from build123d import *

# Parameters (mm, degrees)
F1_DEPTH = 25.4
F3_DEPTH = 12.7
F5_DEPTH = 12.7
F7_DEPTH = 12.7


with BuildPart() as f1:
    # F0 (on Top) → F1 (new body)
    with BuildSketch(Plane.XY):
        Polygon((-12.7, 31.75), (0, 31.75), (0, 0), (12.7, 0), (12.7, 31.75), (25.4, 31.75), (25.4, 57.15), (-12.7, 57.15), align=None)
    extrude(amount=F1_DEPTH)

    # F2 (on face) → F3 (cut)
    with BuildSketch(Plane(origin=(-12.7, 0, 0), x_dir=(0, -1, 0), z_dir=(-1, 0, 0))):
        Polygon((-31.75, 25.4), (-44.45, 25.4), (-31.75, 0), align=None)
    extrude(amount=-F3_DEPTH, mode=Mode.SUBTRACT)

    # F4 (on face) → F5 (cut)
    with BuildSketch(Plane.YZ.offset(25.4)):
        Polygon((31.75, 0), (44.45, 25.4), (31.75, 25.4), align=None)
    extrude(amount=-F5_DEPTH, mode=Mode.SUBTRACT)

    # F6 (on face) → F7 (cut)
    with BuildSketch(Plane(origin=(0, 0, 0), x_dir=(0, -1, 0), z_dir=(-1, 0, 0))):
        Polygon((0, 25.4), (-12.7, 25.4), (0, 0), align=None)
    extrude(amount=-F7_DEPTH, mode=Mode.SUBTRACT)


solid = f1.part
Here's how the part is built. I have some questions about the finished solid (model axes, mm). A direction names the side the tool comes from. Give positions to 0.01 mm unless a question says otherwise; leave off trailing zeros. Loops run counter-clockwise (first coordinate to the right, second up) from the corner with the lowest first, then second, coordinate; pieces in that order, holes last. Notation, with made-up numbers: (88.5, 60.25) -> (108.5, 60.25) arc R24 ccw to (108.5, 87.25) -> close; hole circle Ø9 at (51, -28.75). An arc over 180 degrees is marked (long way). Answer as a JSON object with one key per item and string values. Group by question number.
Item 1: Imagine slicing it at C-C on x = 16.5. Write out the boundary of the cut face in (y, z).
Item 2: Imagine slicing it at D-D on y = 10. Write out the boundary of the cut face in (x, z), then the cut area to 3 significant figures.
Item 3: On a 3-axis mill with a long thin cutter (end or side, diameter ignored), from which of +Z, -Z, +X, -X, +Y, -Y can I reach the whole of each face in a straight line? I mean faces 1 (the flat face through (25.4, 47, 13)), 2 (the flat face through (-6.4, 38.2, 12.9)), 3 (the flat face through (12.7, 22, 13)). Say none if no direction works.
Item 4: Will these pins go through, and if not, where does the flat tip stop? pin 1 (12 mm diameter, centred on y = 10.5, z = 12.5, fed in from +X); pin 2 (3 mm diameter, centred on x = -3.5, z = 5, fed in from -Y); pin 3 (2 mm diameter, centred on x = 10.5, z = 3, fed in from -Y).
Item 5: Imagine slicing it at B-B on y = 38.5. Write out the boundary of the cut face in (x, z), then the cut area to 3 significant figures.
Item 6: Imagine slicing it at A-A on z = 22. Write out the boundary of the cut face in (x, y).
Item 7: I need wall thicknesses on L1, parallel to X at y = 7, z = 10.5; L2, parallel to Y at x = 10.5, z = 15.5; L3, parallel to Y at x = -5, z = 20.75 (3 decimals). Which ranges of each line are inside material? Lowest first, please.
Answer list:
{
 "1": {"outline": "(31.75, 0) -> (57.15, 0) -> (57.15, 25.4) -> (44.45, 25.4) -> close"},
 "2": {"outline": "(0, 0) -> (12.7, 0) -> (12.7, 20) -> (0, 20) -> close", "area": "254 mm2"},
 "3": {"face 1": "+Z, -Z, +X, +Y, -Y", "face 2": "+Z, -X, -Y", "face 3": "+Z, +X, -Y"},
 "4": {"pin 1": "stops at x = 12.7", "pin 2": "stops at y = 33.5", "pin 3": "stops at y = 1"},
 "5": {"outline": "(-12.7, 0) -> (25.4, 0) -> (25.4, 13.5) -> (12.7, 13.5) -> (12.7, 25.4) -> (0, 25.4) -> (0, 13.5) -> (-12.7, 13.5) -> close", "area": "665 mm2"},
 "6": {"outline": "(-12.7, 42.75) -> (0, 42.75) -> (0, 11) -> (12.7, 11) -> (12.7, 42.75) -> (25.4, 42.75) -> (25.4, 57.15) -> (-12.7, 57.15) -> close"},
 "7": {"L1": "x = 0 to 12.7", "L2": "y = 7.75 to 57.15", "L3": "y = 42.125 to 57.15"}
}
